The drawing under review shows one solid part. Ordinate dimensions are in mm from its lowest x, y, z. A direction names the side the tool comes from. Round coordinates to 2 decimals unless told otherwise and drop trailing zeros. Order: outer loops, then holes, each group sorted by start corner. A loop starts at its lowest first (then second) coordinate and runs counter-clockwise, first axis right, second up. Notation, with made-up numbers: M -23.5,42.25 L 35.5,42.25 A17 cw 35.5,51.25 Z; hole C 40,35.25 d8. An arc over 180 degrees is marked long. Use a Markdown table: item, result.
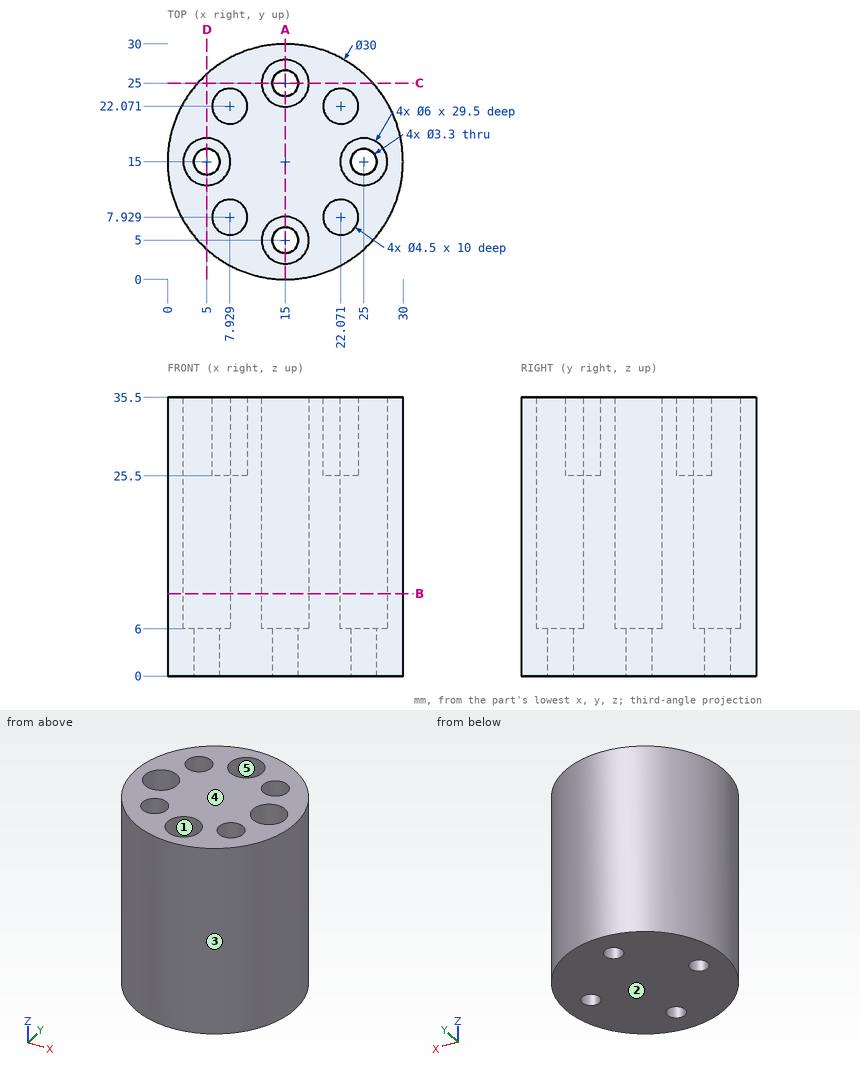
Q1. Wall thickness on line 1 along X through (y, z) = (21.25, 31.5); line 2 along Y through (x, z) = (14.5, 9.5); line 3 along Y through (x, z) = (20.75, 32): over which ranges is each line inside the solid? List them lowest first. Write a range as [from, to].
Determined:
| item | result |
|---|---|
| line 1 | x = [1.36, 5.83], [10.02, 19.98], [24.17, 28.64] |
| line 2 | y = [0.01, 2.04], [7.96, 22.04], [27.96, 29.99] |
| line 3 | y = [1.15, 6.11], [9.75, 20.25], [23.89, 28.85] |
Q2. Add section A-A (x = 15). Write out the cut boundary in (y, z), then the cut area to 3 significant figures.
Determined:
| item | result |
|---|---|
| outline | M 0,0 L 3.35,0 L 3.35,6 L 2,6 L 2,35.5 L 0,35.5 Z; M 6.65,0 L 23.35,0 L 23.35,6 L 22,6 L 22,35.5 L 8,35.5 L 8,6 L 6.65,6 Z; M 26.65,0 L 30,0 L 30,35.5 L 28,35.5 L 28,6 L 26.65,6 Z |
| area | 671 mm^2 |
Q3. Machinability: for the marked faces 1 and 2, which of the approach directions +Z, -Z, +X, -X, +Y, -Y give a long, thin tool a straight path to every point of the face, cutting with its end or side? Answer none if there is none.
Determined:
| item | result |
|---|---|
| face 1 | +Z |
| face 2 | -Z, +X, -X, +Y, -Y |
Q4. Add section C-C (y = 25). Write out the cut boundary in (x, z).
Determined:
| item | result |
|---|---|
| outline | M 3.82,0 L 13.35,0 L 13.35,6 L 12,6 L 12,35.5 L 3.82,35.5 Z; M 16.65,0 L 26.18,0 L 26.18,35.5 L 18,35.5 L 18,6 L 16.65,6 Z |
Q5. Clearance check with flat-ended pins moving along their axes: pin 1 (3 mm diameter, centred on y = 4, z = 22.5, fed in from -X); pin 2 (12 mm diameter, centred on y = 7, z = 4, fed in from +X); pin 3 (5 mm diameter, centred on x = 22.5, z = 26.5, fed in from -Y). State where each tip first meets the part, or that it passes through.
Determined:
| item | result |
|---|---|
| pin 1 | stops at x = 3.39 |
| pin 2 | stops at x = 29.87 |
| pin 3 | stops at y = 0.86 |
Q6. Add section B-B (z = 10.5). Write out the cut boundary in (x, y), then the cut area to 3 significant figures.
Determined:
| item | result |
|---|---|
| outline | C 15,15 d30; hole C 5,15 d6; hole C 15,5 d6; hole C 15,25 d6; hole C 25,15 d6 |
| area | 594 mm^2 |
Q7. Draft analysis for pull direction Y (two halves, no side actions). For the marked faces 3, 4 and 5, state which applies: pulls with the +Y half, pulls with the -Y half, needs draft (parallel to the pull), parting line crosses it, or undercut.
Determined:
| item | result |
|---|---|
| face 3 | parting line crosses it |
| face 4 | needs draft |
| face 5 | undercut |
